Autodesk Inventor part; units mm, degrees
ref_plane "YZ Plane" through (0, 0, 0) normal (1, 0, 0) x (0, 1, 0)
ref_plane "XZ Plane" through (0, 0, 0) normal (0, 1, 0) x (-1, 0, 0)
ref_plane "XY Plane" through (0, 0, 0) normal (0, 0, 1) x (1, 0, 0)
sketch "Skizze1" plane through (0, 0, 0) normal (0, 0, 1) x (1, 0, 0)
  line L0 (-2.15, 4.15) -> (2.15, 4.15)
  line L1 (4.15, 2.15) -> (4.15, -2.15)
  line L2 (2.15, -4.15) -> (-2.15, -4.15)
  line L3 (-4.15, -2.15) -> (-4.15, 2.15)
  arc A0 (-2.15, 4.15) -> (-4.15, 2.15) centre (-2.15, 2.15) ccw
  arc A1 (4.15, 2.15) -> (2.15, 4.15) centre (2.15, 2.15) ccw
  arc A2 (2.15, -4.15) -> (4.15, -2.15) centre (2.15, -2.15) ccw
  arc A3 (-4.15, -2.15) -> (-2.15, -4.15) centre (-2.15, -2.15) ccw
  line L4 (-2.15, 2.15) -> (2.15, -2.15) construction
  line L5 (2.15, 2.15) -> (-2.15, -2.15) construction
  point P0 (0, 0)
  dimension "d0" = 2
  dimension "d1" = 8.3
extrude "Extrusion1" add sketch "Skizze1" along normal blind 3
sketch "Skizze2" plane through (0, 0, 3) normal (0, 0, 1) x (1, 0, 0)
  circle A0 centre (0, 0) radius 2.5
  circle A1 centre (0, 0) radius 3
  dimension "d4" = 5
  dimension "d22" = 6
extrude "Extrusion2" add sketch "Skizze2" along normal blind 12 contours A0
chamfer "Fase1" distance 0.5 angle 45 1 edges at (-2.5, 0, 15)
thread "Gewinde2"
extrude "Extrusion3" add sketch "Skizze2" along normal blind 6.2
sketch "Skizze4" plane through (0, 0, 0) normal (0, 0, -1) x (-1, 0, 0)
  point P0 (0, 0)
  point P1 (0, 0)
hole "Bohrung2" [suppressed]
hole "Bohrung3" at (0, 0, 0) direction (0, 0, 1) diameter 3 depth 10 tip angle 118
chamfer "Fasen2" distance 0.1 angle 45 2 edges at (-3, 0, 9.2) (0, -1.5, 0)
chamfer "Fasen3" [suppressed]
properties part number "RadadapterCLOSED"
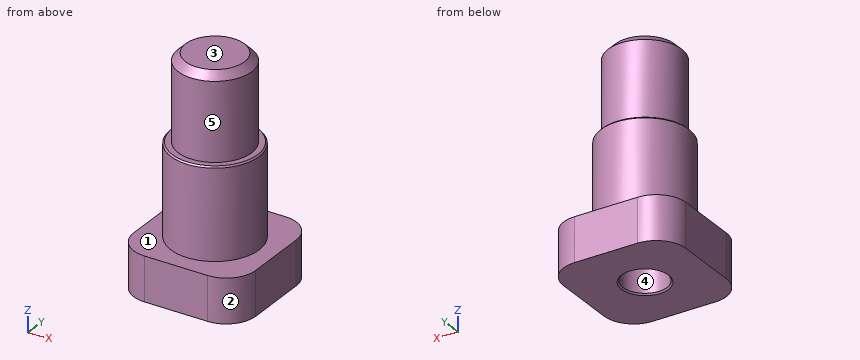
The model under review builds one solid part; all positions refer to its coordinate system, in mm. Face numbers are marked on the shaded views. A direction names the side the tool comes from. Coordinates: 2 decimals unless noted, no trailing zeros. Write each loop counter-clockwise with the first axis right and the second up, starting at its lowest first coordinate (ties: lowest second). Pieces come first, ordered by that corner, then holes. Notation, with made-up numbers: (73, 3) - (103, 3) arc R12 cw to (103, 18) - close; hole circle Ø2 at (60.5, -21.75). An arc over 180 degrees is marked (long way). Answer in a Markdown table with one row per item. Add a question column.
Q1. For the marked faces 1 and 2, list the 3-axis set-ups (+Z, -Z, +X, -X, +Y, -Y) from which the entire face can be reached by the end or side of a thin tool; tool diameter is ignored.
Q2. Consider section B-B on y = 3.25. Give the boundary of the cut face in (x, z), then the cut area to 3 significant figures.
Q3. To check wall thickness, follow line 1 along Y through (x, z) = (0, 2.5); line 2 along Y through (x, z) = (0, 7.75); line 3 along X through (y, z) = (2, 13). State the ranges of each line that lie inside material, in increasing order. Write a range as from..to.
Q4. Draft analysis for pull direction Y (two halves, no side actions). For the marked faces 3, 4 and 5, state which applies: +Y half, -Y half, draft (parallel to the pull), parting line (faces both ways), or undercut.
Q5. Clearance check with flat-ended pins moving along their axes: pin 1 (2 mm diameter, centred on x = -0.5, z = 12, fed in from -Y); pin 2 (1 mm diameter, centred on x = -2.5, z = 12, fed in from +Y). State where each tip first meets the part, or that it passes through.
Q6. Consider section C-C on z = 4.25. Give the boundary of the cut face in (x, y).
Q7. Consider section A-A on z = 1. Give the boundary of the cut face in (x, y).
Answers below:
| question | item | result |
|---|---|---|
| 1 | face 1 | +Z |
| 1 | face 2 | +Z, -Z, +X, -Y |
| 2 | outline | (-3.82, 0) - (3.82, 0) - (3.82, 3) - (-3.82, 3) - close |
| 2 | area | 22.9 mm² |
| 3 | line 1 | -4.15..-1.5, 1.5..4.15 |
| 3 | line 2 | -3..-1.5, 1.5..3 |
| 3 | line 3 | -1.5..1.5 |
| 4 | face 3 | draft |
| 4 | face 4 | undercut |
| 4 | face 5 | parting line |
| 5 | pin 1 | y = -2.5 |
| 5 | pin 2 | y = 1.5 |
| 6 | outline | circle Ø6 at (0, 0); hole circle Ø3 at (0, 0) |
| 7 | outline | (-4.15, -2.15) arc R2 ccw to (-2.15, -4.15) - (2.15, -4.15) arc R2 ccw to (4.15, -2.15) - (4.15, 2.15) arc R2 ccw to (2.15, 4.15) - (-2.15, 4.15) arc R2 ccw to (-4.15, 2.15) - close; hole circle Ø3 at (0, 0) |
